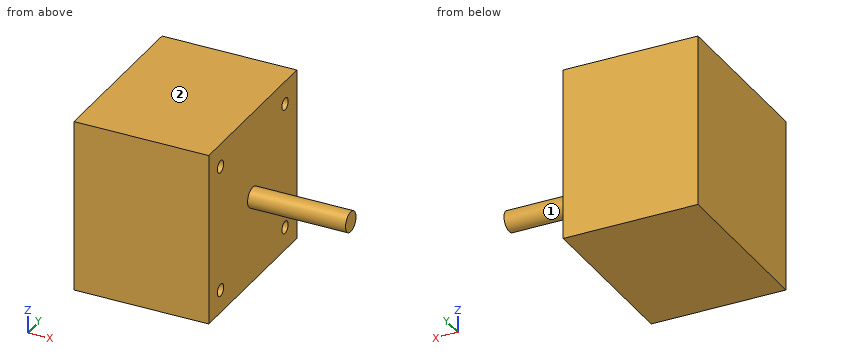
```python
from build123d import *

# Parameters (mm, degrees)
SKETCH_W     = 33
SKETCH_H     = 42.3
PAD_DEPTH    = 21.15
SKETCH001_R  = 2.5
PAD001_DEPTH = 24
SKETCH002_R  = 1.5
POCKET_DEPTH = 4.5


with BuildPart() as part:
    # Sketch → Pad (new body, symmetric)
    with BuildSketch(Plane.XY):
        Rectangle(SKETCH_W, SKETCH_H)
    extrude(amount=PAD_DEPTH, both=True)

    # Sketch001 (on Face1 of Pad) → Pad001 (join)
    with BuildSketch(Plane.YZ.offset(16.5)):
        Circle(SKETCH001_R)
    extrude(amount=PAD001_DEPTH)

    # Sketch002 (on Face1 of Pad001) → Pocket (cut)
    with BuildSketch(Plane.YZ.offset(16.5)):
        with Locations((-15.5, 15.5)):
            Circle(SKETCH002_R)
        with Locations((15.5, 15.5)):
            Circle(SKETCH002_R)
        with Locations((15.5, -15.5)):
            Circle(SKETCH002_R)
        with Locations((-15.5, -15.5)):
            Circle(SKETCH002_R)
    extrude(amount=-POCKET_DEPTH, mode=Mode.SUBTRACT)


solid = part.part
```
The listing builds one solid part. Answer for the finished solid, in the listing's coordinates (mm). Face numbers are marked on the shaded views. A direction names the side the tool comes from. Coordinates: 2 decimals unless noted, no trailing zeros. Loops run counter-clockwise (first coordinate to the right, second up) from the corner with the lowest first, then second, coordinate; pieces in that order, holes last. Notation, with made-up numbers: (-13, 18.5) - (46, 18.5) arc R29 ccw to (46, 51.5) - close; hole circle Ø8 at (56.5, 48). An arc over 180 degrees is marked (long way). Use a Markdown table: item, result. Add a question column.
1) The part is cut by section A-A, the plane z = 0. Give the vertices of the cut face in (x, y).
2) For the marked faces 1 and 2, determine the directions among +Z, -Z, +X, -X, +Y, -Y from which every point of the face is accessible in a straight line to the end or side of a thin tool.
3) The part is cut by section B-B, the plane y = -15.5. Give the vertices of the cut face in (x, z).
4) Given pin 1 (3 mm diameter, centred on x = 28.5, z = -0.5, fed in from -Y); pin 2 (21 mm diameter, centred on y = -2.5, z = 6, fed in from +X); pin 3 (4 mm diameter, centred on y = -15.5, z = -15.5, fed in from +X); pin 4 (0.9 mm diameter, centred on y = 16, z = 15.5, fed in from +X), each flat-ended and moving along its own axis, determine where each tip first touches the part or whether it passes through.
5) The part is cut by section C-C, the plane x = 14.5. Give the vertices of the cut face in (y, z), and give its area (3 significant figures).
6) Find the intervals of material crossed by line 1 (Z direction, x = 15.55, y = 15.5); line 2 (Z direction, x = 13, y = 15), in increasing order.
Here are the results:
| question | item | result |
|---|---|---|
| 1 | outline | (-16.5, -21.15) - (16.5, -21.15) - (16.5, -2.5) - (40.5, -2.5) - (40.5, 2.5) - (16.5, 2.5) - (16.5, 21.15) - (-16.5, 21.15) - close |
| 2 | face 1 | +X |
| 2 | face 2 | +Z, +X, -X, +Y, -Y |
| 3 | outline | (-16.5, -21.15) - (16.5, -21.15) - (16.5, -17) - (12, -17) - (12, -14) - (16.5, -14) - (16.5, 14) - (12, 14) - (12, 17) - (16.5, 17) - (16.5, 21.15) - (-16.5, 21.15) - close |
| 4 | pin 1 | stops at y = -2.5 |
| 4 | pin 2 | stops at x = 40.5 |
| 4 | pin 3 | stops at x = 16.5 |
| 4 | pin 4 | stops at x = 12 |
| 5 | outline | (-21.15, -21.15) - (21.15, -21.15) - (21.15, 21.15) - (-21.15, 21.15) - close; hole circle Ø3 at (-15.5, -15.5); hole circle Ø3 at (-15.5, 15.5); hole circle Ø3 at (15.5, -15.5); hole circle Ø3 at (15.5, 15.5) |
| 5 | area | 1,760 mm^2 |
| 6 | line 1 | z = -21.15 to -17, -14 to 14, 17 to 21.15 |
| 6 | line 2 | z = -21.15 to -16.91, -14.09 to 14.09, 16.91 to 21.15 |
